Autodesk Inventor part; units mm, degrees
ref_plane "YZ Plane" through (0, 0, 0) normal (1, 0, 0) x (0, 1, 0)
ref_plane "XZ Plane" through (0, 0, 0) normal (0, 1, 0) x (-1, 0, 0)
ref_plane "XY Plane" through (0, 0, 0) normal (0, 0, 1) x (1, 0, 0)
sketch "Sketch1" plane through (0, 0, 0) normal (0, 1, 0) x (-1, 0, 0)
  line L0 (0, 0) -> (-500, 0)
  line L1 (-500, 0) -> (-500, -100)
  line L2 (-500, -100) -> (0, -100)
  line L3 (0, -100) -> (0, 0)
  dimension "d0" = 500
  dimension "d1" = 100
extrude "Extrusion1" add sketch "Sketch1" along normal blind 10
sketch "Sketch2" plane through (0, 10, 0) normal (0, 1, 0) x (1, 0, 0)
  point P0 (0, 0)
sketch "Sketch3" plane through (0, 10, 0) normal (0, 1, 0) x (1, 0, 0)
  circle A0 centre (100, 15) radius 5
  circle A1 centre (400, 15) radius 5
  line L0 (0, 0) -> (500, 0)
  line L1 (500, 0) -> (500, 100)
  line L2 (0, 100) -> (0, 0)
  dimension "d5" = 10
  dimension "d6" = 10
  dimension "d7" = 15
  dimension "d8" = 15
  dimension "d9" = 100
  dimension "d10" = 100
extrude "Extrusion2" cut sketch "Sketch3" against normal blind 10
equation "\"d6\" = d5"
equation "\"d8\" = d7"
equation "\"d10\" = d9"
properties part number "blend_10cm"
Geometry check sheet. Reference: the model listing, model coordinates, mm. Give positions to 0.01 mm unless a question says otherwise; leave off trailing zeros. Write each loop counter-clockwise with the first axis right and the second up, starting at its lowest first coordinate (ties: lowest second). Pieces come first, ordered by that corner, then holes.
1) Cross-section at B-B (z = -15). Record the boundary of the cut face in (x, y), plus the area to 3 significant figures.
Values follow:
outline: (0, 0) - (95, 0) - (95, 10) - (0, 10) - close; (105, 0) - (395, 0) - (395, 10) - (105, 10) - close; (405, 0) - (500, 0) - (500, 10) - (405, 10) - close
area: 4,800 mm2
2) Cross-section at A-A (x = 100). Record the boundary of the cut face in (y, z).
Values follow:
outline: (0, -100) - (10, -100) - (10, -20) - (0, -20) - close; (0, -10) - (10, -10) - (10, 0) - (0, 0) - close
3) Go/stop test with flat-tipped pins: pin 1 Ø6 at (x, y) = (255, 6) entering from +Z; pin 2 Ø9 at (x, z) = (400, -15) entering from -Y. Record where each tip stops, or that it passes through.
Values follow:
pin 1: stops at z = 0
pin 2: passes through
4) Thickness scan on line 1 (X direction, y = 5, z = -15); line 2 (Z direction, x = 100, y = 6). Record the ranges inside material, lowest first.
Values follow:
line 1: x = 0 to 95, 105 to 395, 405 to 500
line 2: z = -100 to -20, -10 to 0
